CAD build for the part. Positions are in the model's coordinates, mm. A direction names the side the tool comes from. Round coordinates to 2 decimals unless told otherwise and drop trailing zeros. Loops run counter-clockwise (first coordinate to the right, second up) from the corner with the lowest first, then second, coordinate; pieces in that order, holes last. Notation, with made-up numbers: M -17,89 L -13,89 A27 cw -13,122 Z; hole C 53,-35 d5. An arc over 180 degrees is marked long. Use one line per item in the form item = value.
from build123d import *

# Parameters (mm, degrees)
SKETCH1_W           = 203.2
SKETCH1_H           = 31.75
BOSS_EXTRUDE1_DEPTH = 3.175
SKETCH2_W           = 6.223
SKETCH2_H           = 3.175
BOSS_EXTRUDE2_DEPTH = 3.175
LPATTERN1_COUNT     = 8
LPATTERN1_PITCH     = 25.4


with BuildPart() as part:
    # Sketch1 → Boss-Extrude1 (new body)
    with BuildSketch(Plane(origin=(0, 0, 0), x_dir=(1, 0, 0), z_dir=(0, 1, 0))):
        Rectangle(SKETCH1_W, SKETCH1_H)
    extrude(amount=BOSS_EXTRUDE1_DEPTH)

    # Sketch2 → Boss-Extrude2 (add)
    with BuildSketch(Plane.XY.offset(15.875)):
        with Locations((88.9, 1.5875)):
            Rectangle(SKETCH2_W, SKETCH2_H)
    boss_extrude2 = extrude(amount=BOSS_EXTRUDE2_DEPTH)

    # LPattern1: Boss-Extrude2 ×8
    with Locations(*[(-i * LPATTERN1_PITCH, 0, 0) for i in range(1, LPATTERN1_COUNT)]):
        add(boss_extrude2)


solid = part.part
1. Probe line 1 along Z through (x, y) = (-71, 0.5) (3 decimals). List the from-to ranges inside material, lowest first. Write a range as from..to.
Completed:
line_1 = -15.875..15.875
2. Cut at A-A on x = 47. Write the cut outline in (y, z) (3 decimals).
Completed:
outline = M 0,-15.875 L 3.175,-15.875 L 3.175,15.875 L 0,15.875 Z
3. Drop flat-ended pins along their axis: P1, Ø1.6, axis at y = 1, z = 18, coming from the -X side; P2, Ø1.6, axis at x = 80.5, y = 1, coming from the +Z side (3 decimals); P3, Ø1.6, axis at y = 1.5, z = 17.5, coming from the +X side. Give the stop position or say it passes through.
Completed:
P1 = -92.01
P2 = 15.875
P3 = 92.01
4. Tool access for faces 1 (the face through (41.212, 2, 17)), 2 (the face through (-97, 2, 15.875)), 3 (the face through (-64, 2, 19.05)), 4 (the face through (97, 2, 15.875)), 5 (the face through (-1, 3.175, 1)): list every direction of +Z, -Z, +X, -X, +Y, -Y with a clear straight run to the whole face (end or side of a thin tool).
Completed:
face_1 = +Z, +Y, -Y
face_2 = +Z, -X, +Y, -Y
face_3 = +Z, +X, -X, +Y, -Y
face_4 = +Z, +X, +Y, -Y
face_5 = +Z, -Z, +X, -X, +Y
5. Pull direction X, two halves, no side cores. Call faces 6 (the face through (-92.011, 2, 17)), 7 (the face through (85.788, 2, 17)), 8 (the face through (-89, 2, 19.05)): +X half, -X half, draft (parallel to the pull), parting line (faces both ways), or undercut.
Completed:
face_6 = -X half
face_7 = undercut
face_8 = draft
